CAD build for the part. Positions are in the model's coordinates, mm. Face numbers are marked on the shaded views. A direction names the side the tool comes from. Round coordinates to 2 decimals unless told otherwise and drop trailing zeros. Loops run counter-clockwise (first coordinate to the right, second up) from the corner with the lowest first, then second, coordinate; pieces in that order, holes last. Notation, with made-up numbers: (57.5, -10) - (66.5, -10) arc R17 ccw to (66.5, 21) - close; hole circle Ø11 at (38, 75). An arc over 180 degrees is marked (long way). Use one line per item in the form item = value.
from build123d import *

# Parameters (mm, degrees)
F0_W     = 24
F0_H     = 24
F0_W_2   = 20
F0_H_2   = 20
F1_DEPTH = 42
F2_W     = 33
F2_H     = 20
F3_DEPTH = 31.3
F4_W     = 24
F4_H     = 2
F4_H_2   = 22
F5_DEPTH = 2
F6_R     = 2.6
F7_DEPTH = 25


with BuildPart() as f1:
    # F0 (on Right) → F1 (new body)
    with BuildSketch(Plane.YZ):
        Rectangle(F0_W, F0_H)
        Rectangle(F0_W_2, F0_H_2, mode=Mode.SUBTRACT)
    extrude(amount=F1_DEPTH)

    # F2 (on face) → F3 (cut)
    with BuildSketch(Plane.XZ.offset(12)):
        with Locations((25.5, 0)):
            Rectangle(F2_W, F2_H)
    extrude(amount=-F3_DEPTH, mode=Mode.SUBTRACT)

    # F4 (on face) → F5 (join)
    with BuildSketch(Plane.YZ.offset(42)):
        with Locations((0, -11)):
            Rectangle(F4_W, F4_H)
        with Locations((0, 1)):
            Rectangle(F4_W, F4_H_2)
    extrude(amount=F5_DEPTH)

    # F6 (on face) → F7 (cut)
    with BuildSketch(Plane.YZ.offset(44)):
        with Locations((0, 5.4)):
            Circle(F6_R)
        with Locations((0, -5.4)):
            Circle(F6_R)
    extrude(amount=-F7_DEPTH, mode=Mode.SUBTRACT)


solid = f1.part
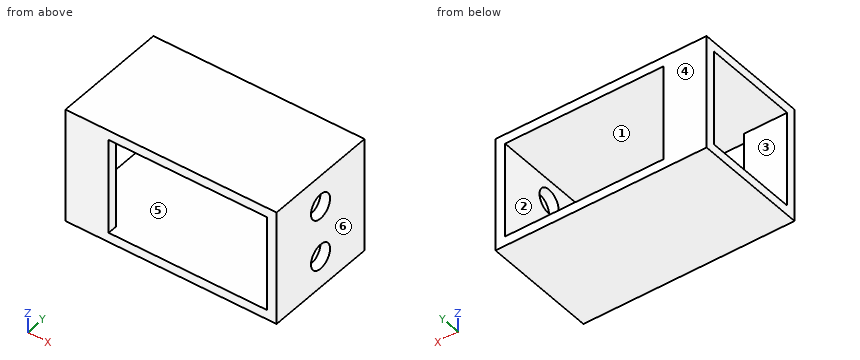
1) Drill centre lines: probe 1 along Z at (x, y) = (42.65, 0); probe 2 along X at (y, z) = (-10.75, 5.75); probe 3 along Z at (x, y) = (29, 3). Where is each one in solid material? Low to high.
Report:
probe_1 = -12 to -8, -2.8 to 2.8, 8 to 12
probe_2 = 0 to 9, 42 to 44
probe_3 = -12 to -10, 10 to 12
2) Slice it at D-D (y = 8.25). Write the cut outline in (x, z), plus the area to 3 significant figures.
Report:
outline = (0, -12) - (44, -12) - (44, 12) - (0, 12) - (0, 10) - (42, 10) - (42, -10) - (0, -10) - close
area = 216 mm^2
3) Two-plate mould, pull along Y, no slides. Class the marked faces 1, 2, 3 and 4: +Y half, -Y half, draft (parallel to the pull), parting line (faces both ways), or undercut.
Report:
face_1 = undercut
face_2 = draft
face_3 = undercut
face_4 = +Y half
4) Slice it at C-C (y = 0). Write the cut outline in (x, z).
Report:
outline = (0, -12) - (44, -12) - (44, -8) - (42, -8) - (42, -10) - (0, -10) - close; (0, 10) - (42, 10) - (42, 8) - (44, 8) - (44, 12) - (0, 12) - close; (42, -2.8) - (44, -2.8) - (44, 2.8) - (42, 2.8) - close
5) Tool access for the marked faces 5 and 6: list every direction of +Z, -Z, +X, -X, +Y, -Y with a clear straight run to the whole face (end or side of a thin tool).
Report:
face_5 = none
face_6 = +Z, -Z, +X, +Y, -Y
6) Slice it at A-A (z = 5.4). Write the cut outline in (x, y), plus the area to 3 significant figures.
Report:
outline = (0, -12) - (9, -12) - (9, -10) - (0, -10) - close; (0, 10) - (9, 10) - (9, 12) - (0, 12) - close; (42, -12) - (44, -12) - (44, -2.6) - (42, -2.6) - close; (42, 2.6) - (44, 2.6) - (44, 12) - (42, 12) - close
area = 73.6 mm^2
7) Slice it at B-B (x = 34.5). Write the cut outline in (y, z).
Report:
outline = (-12, -12) - (12, -12) - (12, -10) - (-12, -10) - close; (-12, 10) - (12, 10) - (12, 12) - (-12, 12) - close
8) Flat gauge pin, fed straight in: pin 1 (8.5 mm diameter, centred on y = 0, z = -5.4, fed in from -X). Where does the tip first touch, or does it go through?
Report:
pin_1 = 42
